Could you check a few things on this model? Use its own coordinates, in mm. Give positions to 0.01 mm unless a question says otherwise; leave off trailing zeros. Order: outer loops, then holes, each group sorted by start corner. A loop starts at its lowest first (then second) coordinate and runs counter-clockwise, first axis right, second up. Notation, with made-up numbers: (84.5, -3.5) -> (104.5, -3.5) arc R22 cw to (104.5, 33.5) -> close; hole circle Ø2 at (20.25, 87). An arc over 180 degrees is marked (long way). One line per item, written item: value.
```python
from build123d import *

# Parameters (mm, degrees)
ESQUISSE1_W        = 8
ESQUISSE1_H        = 10
ESQUISSE1_R        = 1.5
BOSS_EXTRU_1_DEPTH = 5


with BuildPart() as part:
    # Esquisse1 → Boss.-Extru.1 (new body)
    with BuildSketch(Plane.XY):
        Rectangle(ESQUISSE1_W, ESQUISSE1_H)
        with Locations((0, 2.5)):
            Circle(ESQUISSE1_R, mode=Mode.SUBTRACT)
    extrude(amount=BOSS_EXTRU_1_DEPTH)


solid = part.part
```
1) For P1, Ø3.5, axis at x = 0, y = 2.5, coming from the -Z side, with a flat end and sliding along its axis, tell me the tip position at first contact or that it passes through.
Answer below:
P1: stops at z = 0
2) Suppose I cut it at A-A, the plane y = 2.5. Write out the boundary of the cut face in (x, z).
Answer below:
outline: (-4, 0) -> (-1.5, 0) -> (-1.5, 5) -> (-4, 5) -> close; (1.5, 0) -> (4, 0) -> (4, 5) -> (1.5, 5) -> close
3) If I drill on line 1 along Y through (x, z) = (0, 3.65); line 2 along X through (y, z) = (2, 4.55); line 3 along Y through (x, z) = (-0.75, 2.25), over which ranges is the centre line in solid material (lowest first)?
Answer below:
line 1: y = -5 to 1, 4 to 5
line 2: x = -4 to -1.41, 1.41 to 4
line 3: y = -5 to 1.2, 3.8 to 5
4) Suppose I cut it at B-B, the plane x = 0.25. Write out the boundary of the cut face in (y, z), then the cut area to 3 significant figures.
Answer below:
outline: (-5, 0) -> (1.02, 0) -> (1.02, 5) -> (-5, 5) -> close; (3.98, 0) -> (5, 0) -> (5, 5) -> (3.98, 5) -> close
area: 35.2 mm2
5) We'd pull the mould along X, two halves only. Please class faces 1 (the flat face through (0, 0, 5)), 2 (the flat face through (-4, 0, 2)), 3 (the cylindrical face through (0, 1, 2)): +X half, -X half, draft (parallel to the pull), parting line (faces both ways), or undercut.
Answer below:
face 1: draft
face 2: -X half
face 3: undercut
6) Suppose I cut it at C-C, the plane z = 1.85. Write out the boundary of the cut face in (x, y), then the cut area to 3 significant figures.
Answer below:
outline: (-4, -5) -> (4, -5) -> (4, 5) -> (-4, 5) -> close; hole circle Ø3 at (0, 2.5)
area: 72.9 mm2
